from build123d import *

# Parameters (mm, degrees)
F1_DEPTH = 67
F2_R     = 10
F3_SIZE  = 5


with BuildPart() as f1:
    # F0 (on Front) → F1 (new body)
    with BuildSketch(Plane.XZ):
        Polygon((0, 0), (0, 66), (-91, 66), (-12.957165, 240.985362), (-79.623835, 240.985362), (-187.10243, 0), align=None)
    extrude(amount=F1_DEPTH)

    # F2
    f2_edges = [f1.edges().sort_by_distance(p)[0] for p in [
        (-187.10243, -33.5, 0),
    ]]
    fillet(f2_edges, radius=F2_R)

    # F3
    f3_edges = [f1.edges().sort_by_distance(p)[0] for p in [
        (-51.978583, -67, 153.492681),
        (-51.978583, 0, 153.492681),
        (-130.224831, 0, 127.52929),
        (-130.224831, -67, 127.52929),
        (-45.5, 0, 66),
        (-45.5, -67, 66),
    ]]
    chamfer(f3_edges, length=F3_SIZE)


solid = f1.part
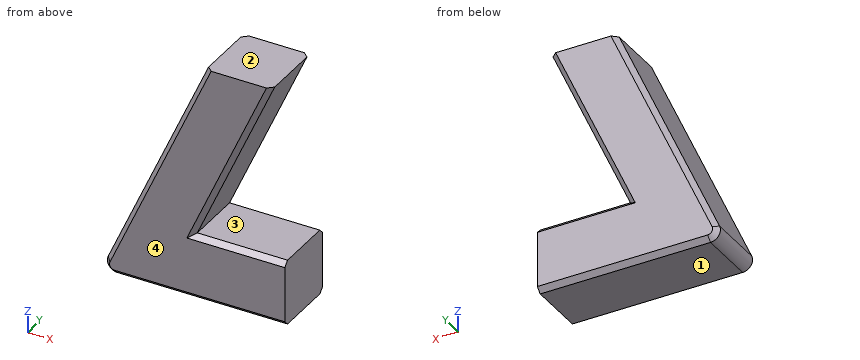
Verification items for the finished model (mm, model axes). Face numbers are marked on the shaded views. Round coordinates to 2 decimals unless told otherwise and drop trailing zeros. Loops run counter-clockwise (first coordinate to the right, second up) from the corner with the lowest first, then second, coordinate; pieces in that order, holes last. Notation, with made-up numbers: (6.25, 2) - (20.25, 2) arc R9 ccw to (20.25, 11) - close; hole circle Ø9 at (-10.75, -3). An arc over 180 degrees is marked (long way). Use a Markdown table: item, result. Add a question column.
1. Section check D-D, the plane z = 19. Record the boundary of the cut face in (x, y), plus the area to 3 significant figures.
2. Section check C-C, the plane z = 133. Record the boundary of the cut face in (x, y), plus the area to 3 significant figures.
3. Thickness scan on probe 1 along Z at (x, y) = (-34, -57); probe 2 along Z at (x, y) = (-10, -60.5); probe 3 along Z at (x, y) = (-62, -60.5). Record the ranges inside material, lowest first. Write a range as [from, to].
4. Section check B-B, the plane x = -154. Record the boundary of the cut face in (y, z), plus the area to 3 significant figures.
5. Gauge pin test, flat ends, axial feed: pin 1 (12 mm diameter, centred on x = -51, z = 147.5, fed in from +Y); pin 2 (6 mm diameter, centred on x = -139.5, y = -41, fed in from +Z); pin 3 (1.5 mm diameter, centred on y = -28, z = 134.5, fed in from +X); pin 4 (3 mm diameter, centred on y = -49, z = 25, fed in from +X). Record the tip position at first contact, or that the pin passes through.
6. Section check A-A, the plane y = -22.5. Record the boundary of the cut face in (x, z).
7. Release check for a two-part mould opening along Z. For the marked faces 1, 2, 3 and 4 record: released by +Z, released by -Z, zero draft, split by the parting line, or undercut.
Checks:
| question | item | result |
|---|---|---|
| 1 | outline | (-178.63, -62) - (-173.15, -67) - (0, -67) - (0, 0) - (-173.15, 0) - (-178.63, -5) - close |
| 1 | area | 11,900 mm^2 |
| 2 | outline | (-127.78, -62) - (-122.31, -67) - (-66.59, -67) - (-61.12, -62) - (-61.12, -5) - (-66.59, 0) - (-122.31, 0) - (-127.78, -5) - close |
| 2 | area | 4,410 mm^2 |
| 3 | probe 1 | z = [0, 66], [193.8, 240.99] |
| 3 | probe 2 | z = [0, 66] |
| 3 | probe 3 | z = [0, 66], [131.02, 240.99] |
| 4 | outline | (-67, 5) - (-62, 0) - (-5, 0) - (0, 5) - (0, 61.95) - (-5, 74.22) - (-62, 74.22) - (-67, 61.95) - close |
| 4 | area | 4,890 mm^2 |
| 5 | pin 1 | stops at y = -2.33 |
| 5 | pin 2 | stops at z = 113.46 |
| 5 | pin 3 | stops at x = -60.11 |
| 5 | pin 4 | stops at x = 0 |
| 6 | outline | (-180.83, 14.07) arc R10 ccw to (-171.69, 0) - (0, 0) - (0, 66) - (-91, 66) - (-12.96, 240.99) - (-79.62, 240.99) - close |
| 7 | face 1 | released by -Z |
| 7 | face 2 | released by +Z |
| 7 | face 3 | undercut |
| 7 | face 4 | zero draft |
